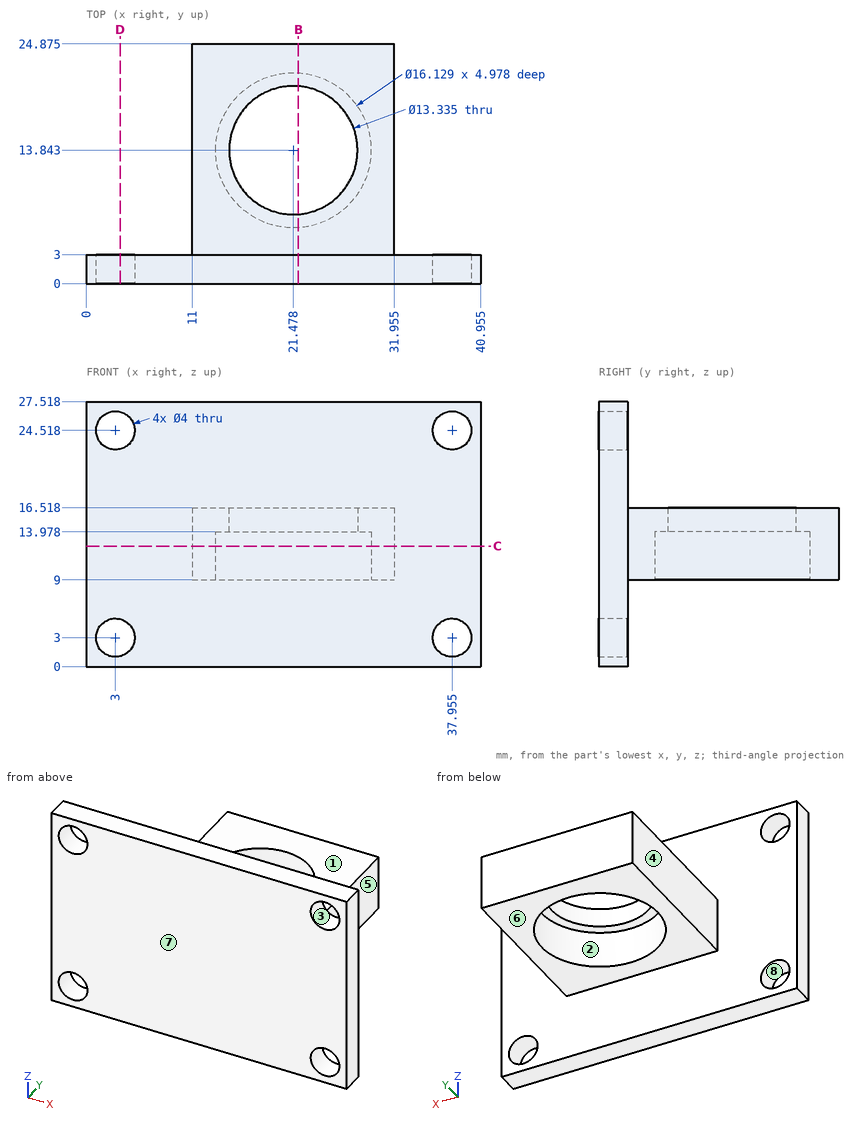
The drawing under review shows one solid part. Ordinate dimensions are in mm from its lowest x, y, z. A direction names the side the tool comes from. Give positions to 0.01 mm unless a question says otherwise; leave off trailing zeros. Order: outer loops, then holes, each group sorted by start corner. A loop starts at its lowest first (then second) coordinate and runs counter-clockwise, first axis right, second up. Notation, with made-up numbers: (-19, -16) -> (1, -16) arc R28 ccw to (1, 16) -> close; hole circle Ø1 at (53, 45.5). An arc over 180 degrees is marked (long way). Write item = value, one per line.
1) For the marked faces 1, 2, 3, 4 and 5, list the 3-axis set-ups (+Z, -Z, +X, -X, +Y, -Y) from which the entire face can be reached by the end or side of a thin tool; tool diameter is ignored.
Findings:
face_1 = +Z, +X, -X, +Y
face_2 = -Z
face_3 = +Y, -Y
face_4 = +Z, -Z, -X, +Y
face_5 = +Z, -Z, +X, +Y
2) Insertion check: pin 1 (6.5 mm diameter, centred on x = 26, y = 17.5, fed in from +Z); pin 2 (2.5 mm diameter, centred on x = 37.96, z = 3, fed in from +Y) (3 decimals); pin 3 (4 mm diameter, centred on y = 10.5, z = 12.5, fed in from +X) (1 decimal); pin 4 (4.5 mm diameter, centred on x = 37.96, z = 24.52, fed in from +Y). Each pin has a flat end and moves straight along its axis. Give the tip position at first contact, or say it passes through.
Findings:
pin_1 = 16.52
pin_2 = through
pin_3 = 32
pin_4 = 3
3) We need section C-C, the plane z = 12.5. Give the boundary of the cut face in (x, y) (1 decimal).
Findings:
outline = (0, 0) -> (41, 0) -> (41, 3) -> (32, 3) -> (32, 24.9) -> (11, 24.9) -> (11, 3) -> (0, 3) -> close; hole circle Ø16.1 at (21.5, 13.8)
4) Draft analysis for pull direction Z (two halves, no side actions). For the marked faces 6, 7 and 8, state which applies: pulls with the +Z half, pulls with the -Z half, needs draft (parallel to the pull), parting line crosses it, or undercut.
Findings:
face_6 = pulls with the -Z half
face_7 = needs draft
face_8 = undercut
5) To check wall thickness, follow L1, parallel to Y at x = 22, z = 8; L2, parallel to X at y = 2.75, z = 24 (1 decimal); L3, parallel to Z at x = 28.5, y = 12.5. State the ranges of each line that lie inside material, in increasing order. Write a range as from..to.
Findings:
L1 = 0..3
L2 = 0..1.1, 4.9..36, 39.9..41
L3 = 13.98..16.52
6) We need section B-B, the plane x = 22. Give the boundary of the cut face in (y, z) (1 decimal).
Findings:
outline = (0, 0) -> (3, 0) -> (3, 9) -> (5.8, 9) -> (5.8, 14) -> (7.2, 14) -> (7.2, 16.5) -> (3, 16.5) -> (3, 27.5) -> (0, 27.5) -> close; (20.5, 14) -> (21.9, 14) -> (21.9, 9) -> (24.9, 9) -> (24.9, 16.5) -> (20.5, 16.5) -> close
7) We need section D-D, the plane x = 3.5. Give the boundary of the cut face in (y, z) (1 decimal).
Findings:
outline = (0, 0) -> (3, 0) -> (3, 1.1) -> (0, 1.1) -> close; (0, 4.9) -> (3, 4.9) -> (3, 22.6) -> (0, 22.6) -> close; (0, 26.5) -> (3, 26.5) -> (3, 27.5) -> (0, 27.5) -> close
